from build123d import *

# Parameters (mm, degrees)
SKETCH_1_W                       = 100
SKETCH_1_H                       = 40
EXTRUDE_1_DEPTH                  = 8
HOLE_WIZARD_M3_2_D               = 2.5
HOLE_WIZARD_M3_2_DEPTH           = 21.5
HOLE_WIZARD_M3_2_TIP             = 0.751075774
HOLE_WIZARD_M3_2_ON_FACE_2_D     = 2.5
HOLE_WIZARD_M3_2_ON_FACE_2_DEPTH = 21.5
HOLE_WIZARD_M3_2_ON_FACE_2_TIP   = 0.751075774
FILLET_1_R                       = 5


with BuildPart() as part:
    # 草图1 → 凸台-拉伸1 (new body)
    with BuildSketch(Plane(origin=(0, 0, 0), x_dir=(1, 0, 0), z_dir=(0, 1, 0))):
        Rectangle(SKETCH_1_W, SKETCH_1_H)
        with BuildLine():
            Line((-40.5, 15.8), (-24.5, 15.8))
            ThreePointArc((-24.5, 15.8), (-22.2, 13.5), (-24.5, 11.2))
            Line((-24.5, 11.2), (-40.5, 11.2))
            ThreePointArc((-40.5, 11.2), (-42.8, 13.5), (-40.5, 15.8))
        make_face(mode=Mode.SUBTRACT)
        with BuildLine():
            Line((-40.5, -11.2), (-24.5, -11.2))
            ThreePointArc((-24.5, -11.2), (-22.2, -13.5), (-24.5, -15.8))
            Line((-24.5, -15.8), (-40.5, -15.8))
            ThreePointArc((-40.5, -15.8), (-42.8, -13.5), (-40.5, -11.2))
        make_face(mode=Mode.SUBTRACT)
        with BuildLine():
            Line((40.5, 15.8), (24.5, 15.8))
            ThreePointArc((24.5, 15.8), (22.2, 13.5), (24.5, 11.2))
            Line((24.5, 11.2), (40.5, 11.2))
            ThreePointArc((40.5, 11.2), (42.8, 13.5), (40.5, 15.8))
        make_face(mode=Mode.SUBTRACT)
        with BuildLine():
            Line((40.5, -11.2), (24.5, -11.2))
            ThreePointArc((24.5, -11.2), (22.2, -13.5), (24.5, -15.8))
            Line((24.5, -15.8), (40.5, -15.8))
            ThreePointArc((40.5, -15.8), (42.8, -13.5), (40.5, -11.2))
        make_face(mode=Mode.SUBTRACT)
    extrude(amount=EXTRUDE_1_DEPTH)

    # M3 螺纹孔2
    with Locations(Plane(origin=(-22.5, 8, 0), x_dir=(0, 0, 1), z_dir=(0, 1, 0))):
        with Locations((0, 0), (0, 45), (0, 22.5)):
            Hole(HOLE_WIZARD_M3_2_D / 2, depth=HOLE_WIZARD_M3_2_DEPTH)
            with Locations((0, 0, -(HOLE_WIZARD_M3_2_DEPTH + HOLE_WIZARD_M3_2_TIP / 2))):  # 118° drill point
                Cone(0, HOLE_WIZARD_M3_2_D / 2, HOLE_WIZARD_M3_2_TIP, mode=Mode.SUBTRACT)

    # M3 螺纹孔2 on face 2
    with Locations(Plane(origin=(0, 0, 0), x_dir=(0, 0, -1), z_dir=(0, -1, 0))):
        with Locations((0, 0)):
            Hole(HOLE_WIZARD_M3_2_ON_FACE_2_D / 2, depth=HOLE_WIZARD_M3_2_ON_FACE_2_DEPTH)
            with Locations((0, 0, -(HOLE_WIZARD_M3_2_ON_FACE_2_DEPTH + HOLE_WIZARD_M3_2_ON_FACE_2_TIP / 2))):  # 118° drill point
                Cone(0, HOLE_WIZARD_M3_2_ON_FACE_2_D / 2, HOLE_WIZARD_M3_2_ON_FACE_2_TIP, mode=Mode.SUBTRACT)

    # 圆角1
    fillet_1_edges = [part.edges().sort_by_distance(p)[0] for p in [
        (50, 4, 20),
        (-50, 4, 20),
        (-50, 4, -20),
        (50, 4, -20),
    ]]
    fillet(fillet_1_edges, radius=FILLET_1_R)


solid = part.part
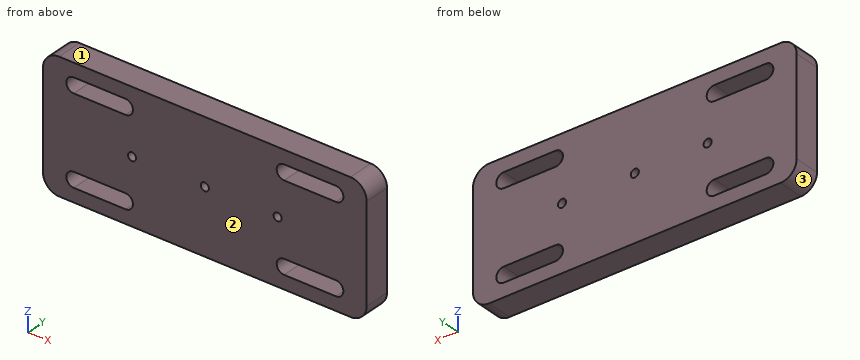
Work out the finished part from the listing and answer in its coordinate system (mm). Face numbers are marked on the shaded views. Round coordinates to 2 decimals unless told otherwise and drop trailing zeros. Write each loop counter-clockwise with the first axis right and the second up, starting at its lowest first coordinate (ties: lowest second). Pieces come first, ordered by that corner, then holes. Notation, with made-up numbers: (-13, 38.25) -> (3, 38.25) arc R26 ccw to (3, 61.25) -> close; hole circle Ø1 at (23, -8.5). An arc over 180 degrees is marked (long way). Write each question's results on one line, items separated by ' | '.
Item 1: A cutting plane is placed at C-C, the plane z = 0. Determine the outline of the cut face in (x, y), plus the area to 3 significant figures.
Result set:
outline: (-50, 0) -> (-23.75, 0) -> (-23.75, 8) -> (-50, 8) -> close; (-21.25, 0) -> (-1.25, 0) -> (-1.25, 8) -> (-21.25, 8) -> close; (1.25, 0) -> (21.25, 0) -> (21.25, 8) -> (1.25, 8) -> close; (23.75, 0) -> (50, 0) -> (50, 8) -> (23.75, 8) -> close | area: 740 mm^2
Item 2: A cutting plane is placed at A-A, the plane x = 39.5. Determine the outline of the cut face in (y, z), plus the area to 3 significant figures.
Result set:
outline: (0, -20) -> (8, -20) -> (8, -15.8) -> (0, -15.8) -> close; (0, -11.2) -> (8, -11.2) -> (8, 11.2) -> (0, 11.2) -> close; (0, 15.8) -> (8, 15.8) -> (8, 20) -> (0, 20) -> close | area: 246 mm^2
Item 3: Find the intervals of material crossed by line 1 along Z through (x, y) = (-26.5, 2); line 2 along X through (y, z) = (4.25, 0); line 3 along Z through (x, y) = (0, 6), in increasing order. Write a range as [from, to].
Result set:
line 1: [-20, -15.8], [-11.2, 11.2], [15.8, 20] | line 2: [-50, -23.75], [-21.25, -1.25], [1.25, 21.25], [23.75, 50] | line 3: [-20, -1.25], [1.25, 20]
Item 4: A cutting plane is placed at B-B, the plane z = -13.5. Determine the outline of the cut face in (x, y).
Result set:
outline: (-50, 0) -> (-42.8, 0) -> (-42.8, 8) -> (-50, 8) -> close; (-22.2, 0) -> (22.2, 0) -> (22.2, 8) -> (-22.2, 8) -> close; (42.8, 0) -> (50, 0) -> (50, 8) -> (42.8, 8) -> close
Item 5: The mould has two halves that part along Z. Classify the marked faces 1, 2 and 3: +Z half, -Z half, draft (parallel to the pull), parting line (faces both ways), or undercut.
Result set:
face 1: +Z half | face 2: draft | face 3: -Z half
Item 6: A cutting plane is placed at D-D, the plane x = 0. Determine the outline of the cut face in (y, z).
Result set:
outline: (0, -20) -> (8, -20) -> (8, -1.25) -> (0, -1.25) -> close; (0, 1.25) -> (8, 1.25) -> (8, 20) -> (0, 20) -> close
